For this review, take the finished solid that the model builds, in its own axes (mm). A direction names the side the tool comes from. Coordinates: 2 decimals unless noted, no trailing zeros. Write each loop counter-clockwise with the first axis right and the second up, starting at its lowest first coordinate (ties: lowest second). Pieces come first, ordered by that corner, then holes. Notation, with made-up numbers: (-20.75, -11) - (-9.75, -11) arc R24 cw to (-9.75, 26) - close; hole circle Ø6 at (-33, 26.25). An arc over 180 degrees is marked (long way). Use one line per item in the form item = value. Start each with the question number.
1) Mouldability with a two-part tool opening along Z and no side actions: class faces 3 (the cylindrical face through (-38.5, -1.61, 24.15)), 4 (the flat face through (0, -13, 39)), 5 (the flat face through (-41, -23, 0)) as pulls with the +Z half, pulls with the -Z half, needs draft (parallel to the pull), parting line crosses it, or undercut.
2) We need section B-B (x = -18). Give the boundary of the cut face in (y, z) (3 decimals), plus the area to 3 significant figures.
3) We need section D-D (z = 17.5). Give the boundary of the cut face in (x, y) (3 decimals).
4) For L1, parallel to Y at x = -38, z = 12 (3 decimals); L2, parallel to X at y = -20.75, z = 46.5 (3 decimals); L3, parallel to Z at x = -31, y = -23.25 (3 decimals), list the stretches that pass through material, from the lowest coordinate up. Write a range as from..to.
5) We need section A-A (y = -17.5). Give the boundary of the cut face in (x, z) (3 decimals).
6) Tool access review of faces 1 (the flat face through (-73.025, -13, 39)), 2 (the flat face through (-41, -23, 79.375)): name each direction out of +Z, -Z, +X, -X, +Y, -Y from which nothing blocks a thin tool from reaching the whole face with its end or side.
7) We need section C-C (z = 38.1). Give the boundary of the cut face in (x, y) (3 decimals).
Autodesk Inventor part; units mm, degrees
ref_plane "YZ Plane" through (0, 0, 0) normal (1, 0, 0) x (0, 1, 0)
ref_plane "XZ Plane" through (0, 0, 0) normal (0, 1, 0) x (-1, 0, 0)
ref_plane "XY Plane" through (0, 0, 0) normal (0, 0, 1) x (1, 0, 0)
sketch "Sketch1" plane through (0, 0, 0) normal (0, 0, 1) x (1, 0, 0)
  line L0 (0, 0) -> (-76.2, 0)
  line L1 (-76.2, 0) -> (-76.2, -25.4)
  line L2 (-76.2, -25.4) -> (0, -25.4)
  line L3 (0, -25.4) -> (0, 0)
  line L4 (-73.025, -22.225) -> (-73.025, -3.175)
  line L5 (-73.025, -3.175) -> (-3.175, -3.175)
  line L6 (-3.175, -3.175) -> (-3.175, -22.225)
  line L7 (-3.175, -22.225) -> (-73.025, -22.225)
  dimension "d0" = 76.2
  dimension "d1" = 25.4
  dimension "d2" = 3.175
extrude "Extrusion1" add sketch "Sketch1" along normal blind 79.375
sketch "Sketch2" plane through (-76.2, -25.4, 0) normal (0, -1, 0) x (1, 0, 0)
  circle A0 centre (40.7924, 38.1) radius 14.2875
  line L0 (0, 0) -> (76.2, 0)
  line L1 (76.2, 0) -> (76.2, 79.375)
  dimension "d5" = 28.575
  dimension "d6" = 38.1
  dimension "d7" = 35.4076
extrude "Extrusion2" cut sketch "Sketch2" against normal blind 25.4
properties part number "other end support"
Determined:
q1.face_3 = undercut
q1.face_4 = needs draft
q1.face_5 = pulls with the -Z half
q2.outline = (-25.4, 0) - (-22.225, 0) - (-22.225, 79.375) - (-25.4, 79.375) - close; (-3.175, 0) - (0, 0) - (0, 79.375) - (-3.175, 79.375) - close
q2.area = 504 mm²
q3.outline = (-76.2, -25.4) - (0, -25.4) - (0, 0) - (-76.2, 0) - close; hole (-73.025, -22.225) - (-3.175, -22.225) - (-3.175, -3.175) - (-73.025, -3.175) - close
q4.L1 = -25.4..-22.225, -3.175..0
q4.L2 = -76.2..-73.025, -3.175..0
q4.L3 = 0..24.509, 51.691..79.375
q5.outline = (-76.2, 0) - (-73.025, 0) - (-73.025, 79.375) - (-76.2, 79.375) - close; (-3.175, 0) - (0, 0) - (0, 79.375) - (-3.175, 79.375) - close
q6.face_1 = +Z, -Z
q6.face_2 = +Z, +X, -X, +Y, -Y
q7.outline = (-76.2, -25.4) - (-49.695, -25.4) - (-49.695, -22.225) - (-73.025, -22.225) - (-73.025, -3.175) - (-49.695, -3.175) - (-49.695, 0) - (-76.2, 0) - close; (-21.12, -25.4) - (0, -25.4) - (0, 0) - (-21.12, 0) - (-21.12, -3.175) - (-3.175, -3.175) - (-3.175, -22.225) - (-21.12, -22.225) - close
